Design review of the part built by this model. Coordinates are the model's own, in mm. A direction names the side the tool comes from. Coordinates: 2 decimals unless noted, no trailing zeros. Write each loop counter-clockwise with the first axis right and the second up, starting at its lowest first coordinate (ties: lowest second). Pieces come first, ordered by that corner, then holes. Notation, with made-up numbers: M -35,-26.5 L 11,-26.5 A37 cw 11,9.5 Z; hole C -16,56 d4. An arc over 180 degrees is marked long. Write each question's results on one line, items separated by ' | '. Start each with the question number.
```python
from build123d import *

# Parameters (mm, degrees)
SKETCH1_R               = 3.175
SKETCH1_R_2             = 6.35
BOSS_EXTRUDE1_DEPTH     = 8.73125
CUT_EXTRUDE1_DEPTH      = 16.875
CUT_EXTRUDE1_DEPTH_BACK = 16.875
SKETCH3_R               = 4.7625
SKETCH3_R_2             = 3.175
BOSS_EXTRUDE2_DEPTH     = 6.35
FILLET1_R               = 25.4
FILLET2_R               = 1.27


with BuildPart() as part:
    # Sketch1 → Boss-Extrude1 (new body, symmetric)
    with BuildSketch(Plane.XY):
        with BuildLine():
            Line((-15.801120859, 68.320227273), (-9.101445615, -0.881149091))
            ThreePointArc((-9.101445615, -0.881149091), (0, -9.144), (9.101445615, -0.881149091))
            Line((9.101445615, -0.881149091), (15.801120859, 68.320227273))
            ThreePointArc((15.801120859, 68.320227273), (0, 85.725), (-15.801120859, 68.320227273))
        make_face()
        Circle(SKETCH1_R, mode=Mode.SUBTRACT)
        with Locations((0, 69.85)):
            Circle(SKETCH1_R_2, mode=Mode.SUBTRACT)
    extrude(amount=BOSS_EXTRUDE1_DEPTH, both=True)

    # Sketch2 → Cut-Extrude1 (cut, two sides)
    with BuildSketch(Plane(origin=(0, -0.404650896, 0), x_dir=(0, 0, -1), z_dir=(1, 0, 0))) as cut_extrude1_sk:
        Polygon((-2.38125, 49.674878169), (-2.38125, 86.129650896), (-8.73125, 86.129650896), (-8.73125, 68.724878169), (-8.73125, 25.976355541), align=None)
        Polygon((8.73125, 68.724878169), (8.73125, 86.129650896), (2.38125, 86.129650896), (2.38125, 49.674878169), (8.73125, 25.976355541), align=None)
        Polygon((-2.794, 25.804650896), (-2.794, -8.739349104), (2.794, -8.739349104), (2.794, 25.804650896), (0, 36.232000852), align=None)
    extrude(amount=CUT_EXTRUDE1_DEPTH, mode=Mode.SUBTRACT)
    extrude(cut_extrude1_sk.sketch, amount=-CUT_EXTRUDE1_DEPTH_BACK, mode=Mode.SUBTRACT)

    # Sketch3 → Boss-Extrude2 (add)
    with BuildSketch(Plane.XY.offset(8.73125)):
        Circle(SKETCH3_R)
        Circle(SKETCH3_R_2, mode=Mode.SUBTRACT)
    boss_extrude2 = extrude(amount=-BOSS_EXTRUDE2_DEPTH)

    # Mirror1: Boss-Extrude2 across plane
    add(boss_extrude2.mirror(Plane.XY))

    # Fillet1
    fillet1_edges = [part.edges().sort_by_distance(p)[0] for p in [
        (0, 25.571704645, -8.73125),
        (0, 49.270227273, -2.38125),
        (0, 25.4, 2.794),
        (0, 25.4, -2.794),
        (0, 49.270227273, 2.38125),
        (0, 25.571704645, 8.73125),
    ]]
    fillet(fillet1_edges, radius=FILLET1_R)

    # Fillet2
    fillet2_edges = [part.edges().sort_by_distance(p)[0] for p in [
        (0, 35.827349956, 0),
    ]]
    fillet(fillet2_edges, radius=FILLET2_R)


solid = part.part
```
Item 1: We need section B-B on y = 1. State the section outline as (x, z) points.
Item 2: We need section D-D on z = -5.75. State the section outline as (x, y) points (3 decimals), then the cut area to 3 significant figures.
Item 3: We need section C-C on x = 0. Count the separate pieces of the cut face and the enclosed holes in it, then the cut area to 3 significant figures.
Item 4: Wall thickness on L1, parallel to Z at x = 6, y = 11; L2, parallel to Y at x = 0, z = -0.35 (3 decimals); L3, parallel to X at y = 69.85, z = 0.65 (3 decimals): over which ranges is each line inside the solid? List them lowest first.
Item 5: For faces 1 (the cylindrical face through (0.167, 25.325, 2.583)), 2 (the flat face through (0.171, 29.958, 1.573)), 3 (the cylindrical face through (0.2, 49.3, 2.6)), list the 3-axis set-ups (+Z, -Z, +X, -X, +Y, -Y) from which the entire face can be reached by the end or side of a thin tool; tool diameter is ignored.
Item 6: Draft analysis for pull direction Z (two halves, no side actions). For faces 4 (the flat face through (0, 10, 8.731)), 5 (the flat face through (0, 10, -2.794)), 6 (the flat face through (0, 62, -2.381)), state which applies: released by +Z, released by -Z, zero draft, split by the parting line, or undercut.
Item 7: Insertion check: pin 1 Ø3 at (x, y) = (-1, 1) entering from +Z; pin 2 Ø9.5 at (x, y) = (-7, 72) entering from +Z; pin 3 Ø5 at (y, z) = (10.5, 5) entering from -X; pin 4 Ø16 at (x, y) = (-1.5, 77) entering from -Z. Each pin has a flat end and moves straight along its axis. Give the tip position at first contact, or say it passes through.
Item 8: We need section A-A on y = 69.85. State the section outline as (x, z) points (3 decimals), then the cut area to 3 significant figures.
Answer:
1) outline: M -9.28,-8.73 L -3.01,-8.73 L -3.01,-2.38 L -4.66,-2.38 L -4.66,-2.79 L -9.28,-2.79 Z; M -9.28,2.79 L -4.66,2.79 L -4.66,2.38 L -3.01,2.38 L -3.01,8.73 L -9.28,8.73 Z; M 3.01,-8.73 L 9.28,-8.73 L 9.28,-2.79 L 4.66,-2.79 L 4.66,-2.38 L 3.01,-2.38 Z; M 3.01,2.38 L 4.66,2.38 L 4.66,2.79 L 9.28,2.79 L 9.28,8.73 L 3.01,8.73 Z
2) outline: M -12.74,36.698 L -9.101,-0.881 A9.144 ccw 9.101,-0.881 L 12.74,36.698 Z; hole C 0,0 d6.35 | area: 904 mm^2
3) separate pieces: 4 | enclosed holes: 0 | area: 693 mm^2
4) L1: z = -8.73 to -2.79, 2.79 to 8.73 | L2: y = 32.141 to 63.5, 76.2 to 85.725 | L3: x = -15.875 to -6.35, 6.35 to 15.875
5) face 1: +X, -X | face 2: +X, -X, -Y | face 3: +Z, +X, -X, +Y
6) face 4: released by +Z | face 5: undercut | face 6: released by -Z
7) pin 1: passes through | pin 2: stops at z = 2.38 | pin 3: stops at x = -10.45 | pin 4: stops at z = -2.38
8) outline: M -15.875,-2.381 L -6.35,-2.381 L -6.35,2.381 L -15.875,2.381 Z; M 6.35,-2.381 L 15.875,-2.381 L 15.875,2.381 L 6.35,2.381 Z | area: 90.7 mm^2
